from build123d import *

# Parameters (mm, degrees)
SKETCH1_W           = 156.4
SKETCH1_H           = 86
BOSS_EXTRUDE1_DEPTH = 3.175
SKETCH3_R           = 1.25
SKETCH3_R_2         = 1.524
CUT_EXTRUDE2_DEPTH  = 90.299051647
SKETCH4_W           = 146.78
SKETCH4_H           = 24.86
CUT_EXTRUDE3_DEPTH  = 90.299051647
SKETCH5_R           = 1.6
CUT_EXTRUDE4_DEPTH  = 90.299051647
SKETCH6_W           = 20
SKETCH6_H           = 10
CUT_EXTRUDE5_DEPTH  = 90.299051647
FILLET1_R           = 5


with BuildPart() as part:
    # Sketch1 → Boss-Extrude1 (new body)
    with BuildSketch(Plane(origin=(0, 0, 0), x_dir=(1, 0, 0), z_dir=(0, 1, 0))):
        Rectangle(SKETCH1_W, SKETCH1_H)
    extrude(amount=BOSS_EXTRUDE1_DEPTH)

    # Sketch3 → Cut-Extrude2 (cut, through all)
    with BuildSketch(Plane.XZ):
        with Locations(Location((-22.7, -19, 0), (0, 0, 270))):
            Circle(SKETCH3_R)
        with Locations(Location((-71.7, -19, 0), (0, 0, 270))):
            Circle(SKETCH3_R)
        with Locations(Location((-71.7, 39, 0), (0, 0, 270))):
            Circle(SKETCH3_R)
        with Locations(Location((-22.7, 39, 0), (0, 0, 270))):
            Circle(SKETCH3_R)
        with Locations(Location((72.025, 28.575, 0), (0, 0, 270))):
            Circle(SKETCH3_R_2)
        with Locations(Location((23.765, 28.575, 0), (0, 0, 270))):
            Circle(SKETCH3_R_2)
        with Locations(Location((68.85, -37.465, 0), (0, 0, 270))):
            Circle(SKETCH3_R_2)
        with Locations(Location((26.94, -37.465, 0), (0, 0, 270))):
            Circle(SKETCH3_R_2)
    extrude(amount=-CUT_EXTRUDE2_DEPTH, mode=Mode.SUBTRACT)

    # Sketch4 → Cut-Extrude3 (cut, through all)
    with BuildSketch(Plane.XZ):
        Rectangle(SKETCH4_W, SKETCH4_H)
    extrude(amount=-CUT_EXTRUDE3_DEPTH, mode=Mode.SUBTRACT)

    # Sketch5 → Cut-Extrude4 (cut, through all)
    with BuildSketch(Plane.XZ):
        with Locations(Location((7.5, -25, 0), (0, 0, 270))):
            Circle(SKETCH5_R)
        with Locations(Location((-7.5, -25, 0), (0, 0, 270))):
            Circle(SKETCH5_R)
        with Locations(Location((-7.5, 25, 0), (0, 0, 270))):
            Circle(SKETCH5_R)
        with Locations(Location((7.5, 25, 0), (0, 0, 270))):
            Circle(SKETCH5_R)
    extrude(amount=-CUT_EXTRUDE4_DEPTH, mode=Mode.SUBTRACT)

    # Sketch6 → Cut-Extrude5 (cut, through all)
    with BuildSketch(Plane.XZ):
        with Locations((0, 34)):
            Rectangle(SKETCH6_W, SKETCH6_H)
        with Locations((0, -34)):
            Rectangle(SKETCH6_W, SKETCH6_H)
    extrude(amount=-CUT_EXTRUDE5_DEPTH, mode=Mode.SUBTRACT)

    # Fillet1
    fillet1_edges = [part.edges().sort_by_distance(p)[0] for p in [
        (78.2, 1.5875, 43),
        (-78.2, 1.5875, 43),
        (-78.2, 1.5875, -43),
        (78.2, 1.5875, -43),
    ]]
    fillet(fillet1_edges, radius=FILLET1_R)


solid = part.part
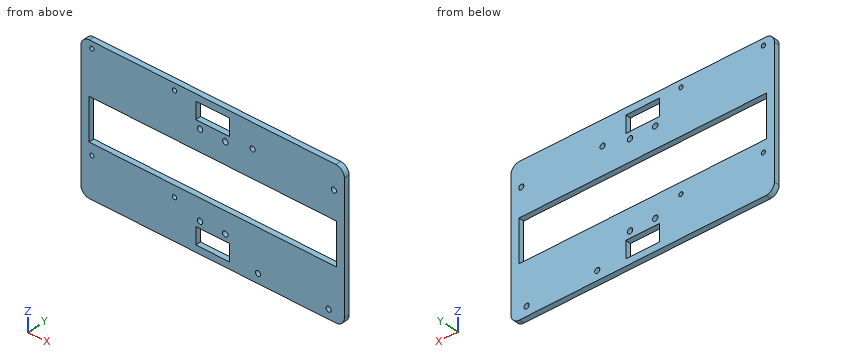
CAD build for the part. Positions are in the model's coordinates, mm. Give positions to 0.01 mm unless a question says otherwise; leave off trailing zeros. Write each loop counter-clockwise with the first axis right and the second up, starting at its lowest first coordinate (ties: lowest second). Pieces come first, ordered by that corner, then holes. Notation, with made-up numbers: (70.25, 48.5) - (74.25, 48.5) arc R35 ccw to (74.25, 85.5) - close; hole circle Ø11 at (41.5, -37.75). An arc over 180 degrees is marked (long way). Answer as CSV lines item,"result".
Q1. Drill centre lines: line 1 (Z direction, x = -22.5, y = 2.1); line 2 (Z direction, x = 68.85, y = 2.4); line 3 (X direction, y = 2.55, z = -19). Where is each one in solid material? Low to high. Write a range as from..to.
Result set:
line 1,"-43..-20.23, -17.77..-12.43, 12.43..37.77, 40.23..43"
line 2,"-43..-38.99, -35.94..-12.43, 12.43..43"
line 3,"-78.2..-72.95, -70.45..-23.95, -21.45..78.2"
Q2. Band-saw the part on D-D (z = 6.5). Give the cut face in (x, y) (3 decimals), and give its area (3 significant figures).
Result set:
outline,"(-78.2, 0) - (-73.39, 0) - (-73.39, 3.175) - (-78.2, 3.175) - close; (73.39, 0) - (78.2, 0) - (78.2, 3.175) - (73.39, 3.175) - close"
area,"30.5 mm²"
Q3. Band-saw the part on A-A (x = 7.5). Give the cut face in (y, z) (3 decimals), and give its area (3 significant figures).
Result set:
outline,"(0, -43) - (3.175, -43) - (3.175, -39) - (0, -39) - close; (0, -29) - (3.175, -29) - (3.175, -26.6) - (0, -26.6) - close; (0, -23.4) - (3.175, -23.4) - (3.175, -12.43) - (0, -12.43) - close; (0, 12.43) - (3.175, 12.43) - (3.175, 23.4) - (0, 23.4) - close; (0, 26.6) - (3.175, 26.6) - (3.175, 29) - (0, 29) - close; (0, 39) - (3.175, 39) - (3.175, 43) - (0, 43) - close"
area,"110 mm²"
Q4. Band-saw the part on C-C (x = 68.85). Give the cut face in (y, z) (3 decimals), and give its area (3 significant figures).
Result set:
outline,"(0, -43) - (3.175, -43) - (3.175, -38.989) - (0, -38.989) - close; (0, -35.941) - (3.175, -35.941) - (3.175, -12.43) - (0, -12.43) - close; (0, 12.43) - (3.175, 12.43) - (3.175, 43) - (0, 43) - close"
area,"184 mm²"
Q5. Band-saw the part on B-B (z = -25). Give the cut face in (x, y) (3 decimals).
Result set:
outline,"(-78.2, 0) - (-9.1, 0) - (-9.1, 3.175) - (-78.2, 3.175) - close; (-5.9, 0) - (5.9, 0) - (5.9, 3.175) - (-5.9, 3.175) - close; (9.1, 0) - (78.2, 0) - (78.2, 3.175) - (9.1, 3.175) - close"
Q6. Flat gauge pin, fed straight in: pin 1 Ø2 at (x, z) = (-71.7, -19) entering from -Y. Where does the tip first touch, or does it go through?
Result set:
pin 1,"through"
